Design review of the part built by this model. Coordinates are the model's own, in mm. A direction names the side the tool comes from. Give positions to 0.01 mm unless a question says otherwise; leave off trailing zeros. Loops run counter-clockwise (first coordinate to the right, second up) from the corner with the lowest first, then second, coordinate; pieces in that order, holes last. Notation, with made-up numbers: M 14.5,60 L 18.5,60 A18 cw 18.5,88 Z; hole C 53,-36 d2. An arc over 180 degrees is marked long. Answer as CSV lines item,"result".
```python
from build123d import *

# Parameters (mm, degrees)
F0_W        = 7
F0_H        = 5
F1_DEPTH    = 1.5
F2_R        = 15
F3_DEPTH    = 2.1
F4_T1_DEPTH = 7
F4_T3_DEPTH = 7


# Not quite as in the source:
# - a fillet or chamfer that OpenCascade refuses, or shapes differently, is made with other operations: its cross-section is extruded or revolved along the edge and cut away or added


with BuildPart() as f1:
    # F0 (on Top) → F1 (new body)
    with BuildSketch(Plane.XY):
        Polygon((0, 8.4325535595), (-17, 8.4325535595), (-17, -46.5674464405), (-10, -46.5674464405), (0, -46.5674464405), (0, -6.5674464405), (-3.25, -6.5674464405), (-3.25, 4.4325535595), (0, 4.4325535595), align=None)
        Polygon((17, 8.4325535595), (0, 8.4325535595), (0, 4.4325535595), (3.25, 4.4325535595), (3.25, -6.5674464405), (0, -6.5674464405), (0, -46.5674464405), (10, -46.5674464405), (17, -46.5674464405), align=None)
        with Locations((13.5, -49.0674464405)):
            Rectangle(F0_W, F0_H)
        with Locations((-13.5, -49.0674464405)):
            Rectangle(F0_W, F0_H)
    extrude(amount=F1_DEPTH)

    # F2
    f2_edges = [f1.edges().sort_by_distance(p)[0] for p in [
        (17, 8.432554, 0.75),
        (-17, 8.432554, 0.75),
    ]]
    fillet(f2_edges, radius=F2_R)

    # F0 (on Top) → F3 (join)
    with BuildSketch(Plane.XY):
        with Locations((13.5, -49.0674464405)):
            Rectangle(F0_W, F0_H)
        with Locations((-13.5, -49.0674464405)):
            Rectangle(F0_W, F0_H)
    extrude(amount=F3_DEPTH)

    # F4: fillet of radius 1 on 2 edges, made by hand

    # F4_s2 → F4_t1 (join)
    with BuildSketch(Plane.YZ.offset(-17)):
        with BuildLine():
            ThreePointArc((-46.5674464405, 2.1), (-46.198653859, 1.6633399735), (-45.6509313015, 1.5))
            Line((-45.6509313015, 1.5), (-46.5674464405, 1.5))
            Line((-46.5674464405, 1.5), (-46.5674464405, 2.1))
        make_face()
    extrude(amount=F4_T1_DEPTH)

    # F4_s4 → F4_t3 (join)
    with BuildSketch(Plane.YZ.offset(10)):
        with BuildLine():
            ThreePointArc((-46.5674464405, 2.1), (-46.198653859, 1.6633399735), (-45.6509313015, 1.5))
            Line((-45.6509313015, 1.5), (-46.5674464405, 1.5))
            Line((-46.5674464405, 1.5), (-46.5674464405, 2.1))
        make_face()
    extrude(amount=F4_T3_DEPTH)


solid = f1.part
```
1. For faces 1 (the flat face through (0, 4.433, 1)), 2 (the flat face through (-14, -51.567, 1)), 3 (the flat face through (0, -46.567, 1)), list the 3-axis set-ups (+Z, -Z, +X, -X, +Y, -Y) from which the entire face can be reached by the end or side of a thin tool; tool diameter is ignored.
Answer block:
face 1,"+Z, -Z"
face 2,"+Z, -Z, +X, -X, -Y"
face 3,"+Z, -Z, -Y"
2. We need section B-B, the plane z = 0.4. Write out the cut boundary in (x, y), plus the area to 3 significant figures.
Answer block:
outline,"M -17,-51.57 L -10,-51.57 L -10,-46.57 L 10,-46.57 L 10,-51.57 L 17,-51.57 L 17,-6.57 A15 ccw 2,8.43 L -2,8.43 A15 ccw -17,-6.57 Z; hole M -3.25,-6.57 L 3.25,-6.57 L 3.25,4.43 L -3.25,4.43 Z"
area,"1,770 mm²"
3. For P1, Ø5, axis at x = 10.5, y = 1, coming from the -Z side; P2, Ø2, axis at x = -4.5, y = 2, coming from the +Z side; P3, Ø1.2, axis at y = 0, z = 0.5, coming from the +X side; P4, Ø1.2, axis at x = -3, z = 0.5, coming from the -Y side, all flat-tipped, find the tip position at first contact; note any pin that passes through.
Answer block:
P1,"z = 0"
P2,"z = 1.5"
P3,"x = 15.76"
P4,"y = -46.57"
4. We need section C-C, the plane x = 13. Write out the cut boundary in (y, z), plus the area to 3 significant figures.
Answer block:
outline,"M -51.57,0 L 3.63,0 L 3.63,1.5 L -45.65,1.5 A1 cw -46.57,2.1 L -51.57,2.1 Z"
area,"86.0 mm²"
5. To check wall thickness, follow L1, parallel to Y at x = -1, z = 0.3; L2, parallel to Z at x = -14, y = -14; L3, parallel to X at y = 1.5, z = 1.3. State the ranges of each line that lie inside material, in increasing order. Write a range as [from, to].
Answer block:
L1,"[-46.57, -6.57], [4.43, 8.43]"
L2,"[0, 1.5]"
L3,"[-14.65, -3.25], [3.25, 14.65]"
6. The part is to be moulded in two halves that separate along Y. For faces 4 (the flat face through (13, -51.567, 1)), 5 (the flat face through (0, -6.567, 1)), 6 (the flat face through (-3.25, -1, 1)), 7 (the flat face through (0, -21, 0)), say which applies: pulls with the +Y half, pulls with the -Y half, needs draft (parallel to the pull), parting line crosses it, or undercut.
Answer block:
face 4,"pulls with the -Y half"
face 5,"undercut"
face 6,"undercut"
face 7,"needs draft"
7. We need section A-A, the plane y = 0.5. Write out the cut boundary in (x, z).
Answer block:
outline,"M -15.23,0 L -3.25,0 L -3.25,1.5 L -15.23,1.5 Z; M 3.25,0 L 15.23,0 L 15.23,1.5 L 3.25,1.5 Z"
8. We need section D-D, the plane y = -12.5. Write out the cut boundary in (x, z).
Answer block:
outline,"M -17,0 L 17,0 L 17,1.5 L -17,1.5 Z"
